Model file for the job. Use its own axes, mm. A direction names the side the tool comes from. Coordinates: 2 decimals unless noted, no trailing zeros. Order: outer loops, then holes, each group sorted by start corner. A loop starts at its lowest first (then second) coordinate and runs counter-clockwise, first axis right, second up. Notation, with made-up numbers: (33, 0) - (38, 0) arc R17 cw to (38, 33) - close; hole circle Ø1 at (66, 79). An arc over 180 degrees is marked (long way). Put each result on its own line as item: value. Start each with the question number.
```python
from build123d import *

# Parameters (mm, degrees)
SKETCH1_W                = 350
SKETCH1_H                = 250
SKETCH1_W_2              = 325.6
SKETCH1_H_2              = 225.61
BOSS_EXTRUDE1_DEPTH      = 120
SKETCH1_2_W              = 325.6
SKETCH1_2_H              = 225.61
BOSS_EXTRUDE2_DEPTH      = 11.6
FILLET1_R                = 10
M8_CLEARANCE_HOLE1_D     = 8.4
M8_CLEARANCE_HOLE1_DEPTH = 8
M8_CLEARANCE_HOLE1_TIP   = 2.5236146


with BuildPart() as part:
    # Sketch1 → Boss-Extrude1 (new body)
    with BuildSketch(Plane(origin=(0, 0, 0), x_dir=(1, 0, 0), z_dir=(0, 1, 0))):
        Rectangle(SKETCH1_W, SKETCH1_H)
        Rectangle(SKETCH1_W_2, SKETCH1_H_2, mode=Mode.SUBTRACT)
    extrude(amount=BOSS_EXTRUDE1_DEPTH)

    # Sketch1<2> → Boss-Extrude2 (add)
    with BuildSketch(Plane(origin=(0, 0, 0), x_dir=(1, 0, 0), z_dir=(0, 1, 0))):
        Rectangle(SKETCH1_2_W, SKETCH1_2_H)
    extrude(amount=BOSS_EXTRUDE2_DEPTH)

    # Fillet1
    fillet1_edges = [part.edges().sort_by_distance(p)[0] for p in [
        (-175, 60, -125),
        (175, 60, -125),
        (175, 60, 125),
        (-175, 60, 125),
    ]]
    fillet(fillet1_edges, radius=FILLET1_R)

    # M8 Clearance Hole1
    with Locations(Plane(origin=(0, 0, 0), x_dir=(-1, 0, 0), z_dir=(0, -1, 0))):
        with Locations((155, -105), (-155, -105), (-155, 105), (155, 105)):
            Hole(M8_CLEARANCE_HOLE1_D / 2, depth=M8_CLEARANCE_HOLE1_DEPTH)
            with Locations((0, 0, -(M8_CLEARANCE_HOLE1_DEPTH + M8_CLEARANCE_HOLE1_TIP / 2))):  # 118° drill point
                Cone(0, M8_CLEARANCE_HOLE1_D / 2, M8_CLEARANCE_HOLE1_TIP, mode=Mode.SUBTRACT)


solid = part.part
```
Item 1: Wall check: line 1 along X through (y, z) = (5, 105); line 2 along Z through (x, y) = (-155, 2); line 3 along Z through (x, y) = (75.5, 106.5) (3 decimals). Give the ranges that are in metal, low to high.
Item 2: 3-axis set-ups, long thin cutter, end or side, ignore diameter. For faces 5 (the face through (-175, 59, 2)), 6 (the face through (-2, 65, -112.805)), 7 (the face through (-158.3, 4.1, 107.6)): which of +Z, -Z, +X, -X, +Y, -Y reach the whole face in a straight line?
Item 3: Slice it at B-B, the plane z = 84. Give the cut face in (x, y), plus the area to 3 significant figures.
Item 4: Slice it at A-A, the plane y = 17. Give the cut face in (x, z) (3 decimals), plus the area to 3 significant figures.
Item 5: Slice it at C-C, the plane x = 107.5. Give the cut face in (y, z) (3 decimals), plus the area to 3 significant figures.
Item 6: Pull direction X, two halves, no side cores. Call faces 1 (the face through (-158.3, 4.1, -102.4)), 2 (the face through (151.7, 4.1, -102.4)), 3 (the face through (-14, 120, 120)), 4 (the face through (-172.15, 60.84, 121.99)): pulls with the +X half, pulls with the -X half, needs draft (parallel to the pull), parting line crosses it, or undercut.
Item 7: Flat gauge pins, fed straight in: pin 1 Ø3 at (x, z) = (133.5, 49) entering from +Y; pin 2 Ø5 at (x, z) = (155, -105) entering from -Y. Where does each tip first touch, or does it go through?
Here are the results:
1. line 1: x = -175 to -159.2, -150.8 to 150.8, 159.2 to 175
1. line 2: z = -125 to -109.2, -100.8 to 100.8, 109.2 to 125
1. line 3: z = -125 to -112.805, 112.805 to 125
2. face 5: +Z, -Z, -X, +Y, -Y
2. face 6: +Y
2. face 7: -Y
3. outline: (-175, 0) - (175, 0) - (175, 120) - (162.8, 120) - (162.8, 11.6) - (-162.8, 11.6) - (-162.8, 120) - (-175, 120) - close
3. area: 6,700 mm^2
4. outline: (-175, -115) arc R10 ccw to (-165, -125) - (165, -125) arc R10 ccw to (175, -115) - (175, 115) arc R10 ccw to (165, 125) - (-165, 125) arc R10 ccw to (-175, 115) - close; hole (-162.8, -112.805) - (162.8, -112.805) - (162.8, 112.805) - (-162.8, 112.805) - close
4. area: 14,000 mm^2
5. outline: (0, -125) - (120, -125) - (120, -112.805) - (11.6, -112.805) - (11.6, 112.805) - (120, 112.805) - (120, 125) - (0, 125) - close
5. area: 5,540 mm^2
6. face 1: undercut
6. face 2: undercut
6. face 3: needs draft
6. face 4: pulls with the -X half
7. pin 1: stops at y = 11.6
7. pin 2: stops at y = 9.02
